CAD build for the part. Positions are in the model's coordinates, mm. A direction names the side the tool comes from. Round coordinates to 2 decimals unless told otherwise and drop trailing zeros. Order: outer loops, then holes, each group sorted by start corner. A loop starts at its lowest first (then second) coordinate and runs counter-clockwise, first axis right, second up. Notation, with made-up numbers: M 39,26 L 88,26 A25 cw 88,43 Z; hole C 84.25,38 d7. An arc over 180 degrees is marked long. Answer as a JSON object with one key per item and string values.
```python
from build123d import *

# Parameters (mm, degrees)
F0_R     = 2
F1_DEPTH = 7
F3_DEPTH = 5.2
F4_R     = 2
F5_DEPTH = 1.75
F7_DEPTH = 1.75


with BuildPart() as f1:
    # F0 (on Top) → F1 (new body)
    with BuildSketch(Plane.XY):
        with BuildLine():
            Line((4.9350217689, -0.0139416518), (19.004955283, 2.4555e-06))
            ThreePointArc((19.004955283, 2.4555e-06), (22.2293780558, 1.1827867006), (23.9300664859, 4.1666666667))
            Line((23.9300664859, 4.1666666667), (26.0782552237, 3.8035564963))
            ThreePointArc((26.0782552237, 3.8035564963), (34.3758111212, 1.3887256489), (32.3801124961, 9.7969376403))
            Line((32.3801124961, 9.7969376403), (23.1300664859, 12.6000024555))
            Line((23.1300664859, 12.6000024555), (11.221314861, 11.6563943987))
            ThreePointArc((11.221314861, 11.6563943987), (5.4972893091, 17.9982805275), (2.4963756955, 9.9996240357))
            Line((2.4963756955, 9.9996240357), (-0.0699335141, 7.9860583482))
            Line((-0.0699335141, 7.9860583482), (-0.0699335141, 4.9860558927))
            ThreePointArc((-0.0699335141, 4.9860558927), (1.3962849714, 1.4487704636), (4.9350217689, -0.0139416518))
        make_face()
        with Locations((30.9300664859, 5.0118209214)):
            Circle(F0_R, mode=Mode.SUBTRACT)
        with Locations((6.4300664859, 13.0860583482)):
            Circle(F0_R, mode=Mode.SUBTRACT)
    extrude(amount=F1_DEPTH)

    # F2 (on face) → F3 (cut)
    with BuildSketch(Plane.XY.offset(7)):
        with BuildLine():
            Line((19.004955283, 7.3360559031), (-0.0699335141, 7.3360559031))
            Line((-0.0699335141, 7.3360559031), (-0.0699335141, 4.9860558927))
            ThreePointArc((-0.0699335141, 4.9860558927), (0.0789501004, 3.7749944518), (0.5167344114, 2.6360558927))
            Line((0.5167344114, 2.6360558927), (19.0047344114, 2.6360558927))
            ThreePointArc((19.0047344114, 2.6360558927), (21.3549552908, 4.985945457), (19.004955283, 7.3360559031))
        make_face()
    extrude(amount=-F3_DEPTH, mode=Mode.SUBTRACT)

    # F4 (on face) → F5 (cut)
    with BuildSketch(Plane.XY):
        with BuildLine():
            Line((-0.064623992, 7.9902242809), (6.5034230268, 8.0865964954))
            ThreePointArc((6.5034230268, 8.0865964954), (9.4470118806, 9.0988236567), (11.221314861, 11.6563943987))
            ThreePointArc((11.221314861, 11.6563943987), (5.4991508888, 17.9986336557), (2.494037584, 10.0026063081))
            ThreePointArc((2.494037584, 10.0026063081), (2.4952063572, 10.0011149504), (2.4963756955, 9.9996240357))
            Line((2.4963756955, 9.9996240357), (-0.064623992, 7.9902242809))
        make_face()
        with Locations((6.4300664859, 13.0860583482)):
            Circle(F4_R, mode=Mode.SUBTRACT)
    extrude(amount=F5_DEPTH, mode=Mode.SUBTRACT)

    # F6 (on face) → F7 (cut)
    with BuildSketch(Plane.XY.offset(7)):
        with BuildLine():
            Line((-0.0699335141, 7.9860583482), (6.5065307879, 8.0866430614))
            ThreePointArc((6.5065307879, 8.0866430614), (8.5828375136, 17.5988819546), (2.4963756955, 9.9996240357))
            Line((2.4963756955, 9.9996240357), (-0.0699335141, 7.9860583482))
        make_face()
    extrude(amount=-F7_DEPTH, mode=Mode.SUBTRACT)


solid = f1.part
```
Item 1: Saw through at A-A on x = 31.5. List the corners of the cut face in (y, z).
Worked answers:
{"outline": "M 0.04,0 L 3.09,0 L 3.09,7 L 0.04,7 Z; M 6.93,0 L 10.06,0 L 10.06,7 L 6.93,7 Z"}
Item 2: Drop flat-ended pins along their axis: pin 1 Ø3 at (x, y) = (3.5, 13.5) entering from +Z; pin 2 Ø4 at (x, z) = (22.5, 1.5) entering from +Y; pin 3 Ø3 at (x, y) = (5.5, 11.5) entering from -Z. Give the stop position or say it passes through.
Worked answers:
{"pin 1": "stops at z = 5.25", "pin 2": "stops at y = 12.6", "pin 3": "stops at z = 1.75"}
Item 3: Saw through at B-B on z = 6.25. List the corners of the cut face in (x, y).
Worked answers:
{"outline": "M -0.07,7.34 L 19,7.34 A2.35 cw 19,2.64 L 0.52,2.64 A5 ccw 4.94,-0.01 L 19,0 A5 ccw 23.93,4.17 L 26.08,3.8 A5 ccw long 32.38,9.8 L 23.13,12.6 L 11.22,11.66 A5 cw 6.51,8.09 L -0.07,7.99 Z; hole C 30.93,5.01 d4"}
Item 4: 3-axis set-ups, long thin cutter, end or side, ignore diameter. For faces 1 (the flat face through (4, 13, 1.75)), 2 (the flat face through (10, 7.336, 4)), 3 (the flat face through (1.231, 9.007, 3.172)), 4 (the flat face through (4, 13, 5.25)): which of +Z, -Z, +X, -X, +Y, -Y reach the whole face in a straight line?
Worked answers:
{"face 1": "-Z, -X, +Y", "face 2": "+Z, -X", "face 3": "+Z, -Z, -X", "face 4": "+Z, -X, +Y"}
Item 5: Saw through at C-C on y = 5.5. List the corners of the cut face in (x, z).
Worked answers:
{"outline": "M -0.07,0 L 28.99,0 L 28.99,7 L 21.3,7 L 21.3,1.8 L -0.07,1.8 Z; M 32.87,0 L 35.91,0 L 35.91,7 L 32.87,7 Z"}
Item 6: Wall check: line 1 along X through (y, z) = (3.5, 3.5); line 2 along X through (y, z) = (5.5, 1); line 3 along Y through (x, z) = (4, 4.25). Give the ranges that are in metal, low to high. Write a range as [from, to].
Worked answers:
{"line 1": "x = [20.83, 23.77], [26.16, 29.62], [32.24, 35.7]", "line 2": "x = [-0.07, 28.99], [32.87, 35.91]", "line 3": "y = [0.07, 2.64], [7.34, 17.46]"}
Item 7: Two-plate mould, pull along Y, no slides. Class faces 5 (the flat face through (27.82, 11.18, 3.45)), 6 (the flat face through (18, 6, 0)), 7 (the flat face through (10, 2.636, 4)): released by +Y, released by -Y, zero draft, split by the parting line, or undercut.
Worked answers:
{"face 5": "released by +Y", "face 6": "zero draft", "face 7": "undercut"}
Item 8: Saw through at D-D on y = 10.5. List the corners of the cut face in (x, z).
Worked answers:
{"outline": "M 2.15,1.75 L 10.71,1.75 L 10.71,0 L 30.06,0 L 30.06,7 L 10.71,7 L 10.71,5.25 L 2.15,5.25 Z"}
